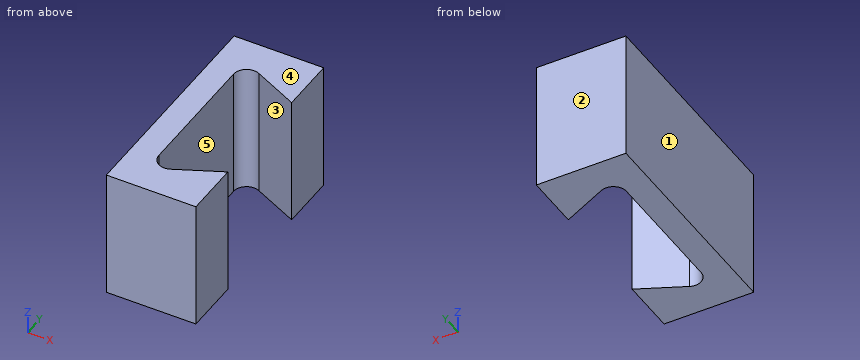
Autodesk Inventor part; units mm, degrees
ref_plane "YZ Plane" through (0, 0, 0) normal (1, 0, 0) x (0, 1, 0)
ref_plane "XZ Plane" through (0, 0, 0) normal (0, 1, 0) x (-1, 0, 0)
ref_plane "XY Plane" through (0, 0, 0) normal (0, 0, 1) x (1, 0, 0)
sketch "Sketch1" plane through (0, 0, 0) normal (0, 0, 1) x (1, 0, 0)
  circle A0 centre (2.8524, -17.9) radius 2
  circle A1 centre (18.8524, -17.9) radius 2
  circle A2 centre (18.8524, 17.9) radius 2
  circle A3 centre (2.8524, 17.9) radius 2
  arc A4 (3.1135, 5.1575) -> (3.0054, 10.8589) centre (-1.0472, 7.9303) ccw
  arc A5 (3.1135, 5.1575) -> (2.4476, 3.9812) centre (10.8524, 0) ccw
  line L0 (2.4476, 3.9812) -> (-1.0195, 5.6235)
  line L1 (-2.4476, 4.7198) -> (-2.4476, -4.7198)
  line L2 (-1.0195, -5.6235) -> (2.4476, -3.9812)
  arc A6 (2.4476, -3.9812) -> (3.1135, -5.1575) centre (10.8524, 0) ccw
  arc A7 (3.0054, -10.8589) -> (3.1135, -5.1575) centre (-1.0472, -7.9303) ccw
  line L3 (-0.3897, -15.5572) -> (3.0054, -10.8589)
  arc A8 (-0.3897, -15.5572) -> (6.4079, -19.7325) centre (2.8524, -17.9) ccw
  arc A9 (15.2968, -19.7325) -> (6.4079, -19.7325) centre (10.8524, -22.0231) ccw
  arc A10 (15.2968, -19.7325) -> (22.0945, -15.5572) centre (18.8524, -17.9) ccw
  line L4 (22.0945, -15.5572) -> (18.6993, -10.8589)
  arc A11 (18.3102, -5.6345) -> (18.6993, -10.8589) centre (22.752, -7.9303) ccw
  line L5 (32.1524, -5.6345) -> (18.3102, -5.6345)
  line L6 (32.1524, 5.6345) -> (32.1524, -5.6345)
  line L7 (32.1524, 5.6345) -> (18.3102, 5.6345)
  arc A12 (18.6993, 10.8589) -> (18.3102, 5.6345) centre (22.752, 7.9303) ccw
  line L8 (18.6993, 10.8589) -> (22.0945, 15.5572)
  arc A13 (22.0945, 15.5572) -> (15.2968, 19.7325) centre (18.8524, 17.9) ccw
  arc A14 (6.4079, 19.7325) -> (15.2968, 19.7325) centre (10.8524, 22.0231) ccw
  arc A15 (6.4079, 19.7325) -> (-0.3897, 15.5572) centre (2.8524, 17.9) ccw
  line L9 (3.0054, 10.8589) -> (-0.3897, 15.5572)
  circle A16 centre (10.8524, 0) radius 1.5
  line L10 (2.2476, 4.2972) -> (-2.6476, 6.616)
  line L11 (-2.6476, 6.616) -> (-2.6476, -6.616)
  line L12 (-2.6476, -6.616) -> (2.2476, -4.2972)
  line L13 (0, 0) -> (10.8524, 0) construction
  line L14 (2.2476, 4.2972) -> (2.2476, 8.616)
  line L15 (2.2476, 8.616) -> (-4.6476, 8.616)
  line L16 (-4.6476, 8.616) -> (-4.6476, -8.616)
  line L17 (-4.6476, -8.616) -> (2.2476, -8.616)
  line L18 (2.2476, -8.616) -> (2.2476, -4.2972)
  arc A17 (-2.4476, -4.7198) -> (-1.0195, -5.6235) centre (-1.4476, -4.7198) ccw
  arc A18 (-1.0195, 5.6235) -> (-2.4476, 4.7198) centre (-1.4476, 4.7198) ccw
  dimension "d0" = 0.2
  dimension "d1" = 0.2
  dimension "d2" = 0.2
  dimension "d3" = 2
  dimension "d4" = 2
extrude "Extrusion1" add sketch "Sketch1" against normal blind 10 contours L10 L11 L12 L18 L17 L16 L15 L14
fillet "Fillet1" radius 1 2 edges at (-2.6476, -6.616, -5) (-2.6476, 6.616, -5)
properties part number "dovetail insert"
The listing builds one solid part. Answer for the finished solid, in the listing's coordinates (mm). Face numbers are marked on the shaded views. A direction names the side the tool comes from. Coordinates: 2 decimals unless noted, no trailing zeros. Order: outer loops, then holes, each group sorted by start corner. A loop starts at its lowest first (then second) coordinate and runs counter-clockwise, first axis right, second up. Notation, with made-up numbers: M 62.25,19.25 L 83.25,19.25 A30 ccw 83.25,53.25 Z; hole C -26,44.25 d7. An arc over 180 degrees is marked long. Answer as a JSON object with one key per item and string values. Group by question number.
1. Section A-A on x = 0 is taken. Write down the section's boundary in (y, z).
2. A tool of negligible diameter and unlimited length cuts with its end or side. For the marked faces 4 and 5, from which of +Z, -Z, +X, -X, +Y, -Y can it reach the whole face along a straight path? Write none if from no direction.
3. Section B-B on y = -5.25 is taken. Write down the section's boundary in (x, z).
4. Determine the mould class of the marked faces 1, 2 and 3 for opening direction Y: released by +Y, released by -Y, zero draft, split by the parting line, or undercut.
5. Section C-C on z = -2.5 is taken. Write down the section's boundary in (x, y).
6. Straight lines are drawn through the part: line 1 (X direction, y = 0.25, z = -7.25); line 2 (Y direction, x = -2, z = -4); line 3 (Y direction, x = 1, z = -7.75). For each, find the intervals that lie inside material, in ascending order.
7. Section D-D on y = 4 is taken. Write down the section's boundary in (x, z).
8. A flat-ended cylindrical pin translates along its axis: P1, Ø3, axis at y = 1.5, z = -6, coming from the +X side. Find the tip coordinate at first contact, or state that the pin passes through.
Values follow:
{
 "1": {"outline": "M -8.62,-10 L -5.36,-10 L -5.36,0 L -8.62,0 Z; M 5.36,-10 L 8.62,-10 L 8.62,0 L 5.36,0 Z"},
 "2": {"face 4": "+Z, +X, -X, +Y, -Y", "face 5": "+Z, -Z"},
 "3": {"outline": "M -4.65,-10 L -2.62,-10 L -2.62,0 L -4.65,0 Z; M 0.24,-10 L 2.25,-10 L 2.25,0 L 0.24,0 Z"},
 "4": {"face 1": "zero draft", "face 2": "released by +Y", "face 3": "undercut"},
 "5": {"outline": "M -4.65,-8.62 L 2.25,-8.62 L 2.25,-4.3 L -1.22,-5.94 A1 cw -2.65,-5.04 L -2.65,5.04 A1 cw -1.22,5.94 L 2.25,4.3 L 2.25,8.62 L -4.65,8.62 Z"},
 "6": {"line 1": "-4.65 to -2.65", "line 2": "-8.62 to -5.97, 5.97 to 8.62", "line 3": "-8.62 to -4.89, 4.89 to 8.62"},
 "7": {"outline": "M -4.65,-10 L -2.65,-10 L -2.65,0 L -4.65,0 Z"},
 "8": {"P1": "x = -2.65"}
}
